The drawing under review shows one solid part. Ordinate dimensions are in mm from its lowest x, y, z. Coordinates: 2 decimals unless noted, no trailing zeros. Loops run counter-clockwise (first coordinate to the right, second up) from the corner with the lowest first, then second, coordinate; pieces in that order, holes last. Notation, with made-up numbers: M -1.5,-6 L 53.5,-6 A29 ccw 53.5,32 Z; hole C -12,84 d2. An arc over 180 degrees is marked long. Put each result on its own line as item: value.
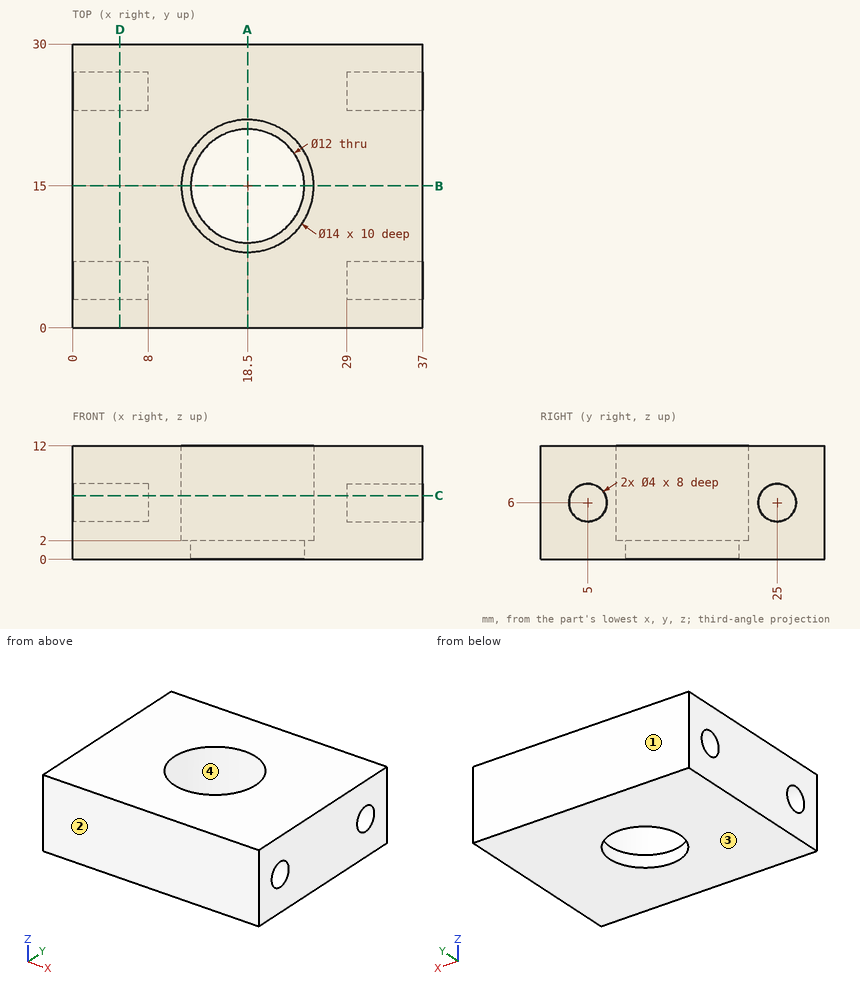
(1) Draft analysis for pull direction Y (two halves, no side actions). For the marked faces 1, 2, 3 and 4, state which applies: +Y half, -Y half, draft (parallel to the pull), parting line (faces both ways), or undercut.
Determined:
face 1: +Y half
face 2: -Y half
face 3: draft
face 4: undercut
(2) For pin 1 (7 mm diameter, centred on x = 15.5, y = 14.5, fed in from +Z); pin 2 (5 mm diameter, centred on y = 5, z = 6, fed in from +X); pin 3 (3 mm diameter, centred on y = 25, z = 6, fed in from +X); pin 4 (1.2 mm diameter, centred on y = 4.5, z = 6, fed in from -X), all flat-tipped, find the tip position at first contact; note any pin that passes through.
Determined:
pin 1: stops at z = 2
pin 2: stops at x = 37
pin 3: stops at x = 29
pin 4: stops at x = 8
(3) Add section A-A (x = 18.5). Write out the cut boundary in (y, z).
Determined:
outline: M 0,0 L 9,0 L 9,2 L 8,2 L 8,12 L 0,12 Z; M 21,0 L 30,0 L 30,12 L 22,12 L 22,2 L 21,2 Z
(4) Add section C-C (z = 6.75). Write out the cut boundary in (x, y).
Determined:
outline: M 0,0 L 37,0 L 37,3.15 L 29,3.15 L 29,6.85 L 37,6.85 L 37,23.15 L 29,23.15 L 29,26.85 L 37,26.85 L 37,30 L 0,30 L 0,26.85 L 8,26.85 L 8,23.15 L 0,23.15 L 0,6.85 L 8,6.85 L 8,3.15 L 0,3.15 Z; hole C 18.5,15 d14
(5) Wall thickness on line 1 along Y through (x, z) = (18.5, 5); line 2 along Z through (x, y) = (5.75, 5); line 3 along X through (y, z) = (10, 8.5): over which ranges is each line inside the solid? List them lowest first. Write a range as [from, to].
Determined:
line 1: y = [0, 8], [22, 30]
line 2: z = [0, 4], [8, 12]
line 3: x = [0, 13.6], [23.4, 37]
(6) Add section B-B (y = 15). Write out the cut boundary in (x, z).
Determined:
outline: M 0,0 L 12.5,0 L 12.5,2 L 11.5,2 L 11.5,12 L 0,12 Z; M 24.5,0 L 37,0 L 37,12 L 25.5,12 L 25.5,2 L 24.5,2 Z
(7) Add section D-D (x = 5). Write out the cut boundary in (y, z), plus the area to 3 significant figures.
Determined:
outline: M 0,0 L 30,0 L 30,12 L 0,12 Z; hole C 5,6 d4; hole C 25,6 d4
area: 335 mm^2
